Work out the finished part from the listing and answer in its coordinate system (mm). A direction names the side the tool comes from. Give positions to 0.01 mm unless a question says otherwise; leave off trailing zeros. Write each loop counter-clockwise with the first axis right and the second up, starting at its lowest first coordinate (ties: lowest second). Pieces come first, ordered by that corner, then holes. Notation, with made-up numbers: (72.25, 68.5) - (89.25, 68.5) arc R10 cw to (89.25, 74.5) - close; hole circle Ø2 at (53.25, 74.25). An arc over 180 degrees is marked (long way). Write item = value, one per line.
from build123d import *

# Parameters (mm, degrees)
F0_W     = 60
F0_H     = 30
F1_DEPTH = 30
F2_W     = 30
F2_H     = 30
F3_DEPTH = 40
F3_TAPER = 7
F4_R     = 7.1976041046
F5_DEPTH = 40


with BuildPart() as f1:
    # F0 (on Front) → F1 (new body)
    with BuildSketch(Plane.XZ):
        with Locations((-30, -15)):
            Rectangle(F0_W, F0_H)
    extrude(amount=F1_DEPTH)

    # F2 (on face) → F3 (join)
    with BuildSketch(Plane.XY):
        with Locations((-15, -15)):
            Rectangle(F2_W, F2_H)
    extrude(amount=F3_DEPTH, taper=F3_TAPER)

    # F4 (on face) → F5 (cut)
    with BuildSketch(Plane.XY.offset(40)):
        with Locations((-15, -13.6708561331)):
            Circle(F4_R)
    extrude(amount=-F5_DEPTH, mode=Mode.SUBTRACT)


solid = f1.part
1. Find section D-D, the plane x = -24. Give the vertices of the cut face in (y, z).
Solution:
outline = (-30, -30) - (0, -30) - (0, 0) - (-4.91, 40) - (-25.09, 40) - (-30, 0) - close
2. A tool of negligible diameter and unlimited length cuts with its end or side. For faces 4 (the flat face through (-45, -15, 0)), 5 (the flat face through (-15, -14, 0)), 6 (the flat face through (-2.42, -14.79, 19.72)), from which of +Z, -Z, +X, -X, +Y, -Y can it reach the whole face along a straight path? Write none if from no direction.
Solution:
face_4 = +Z, -X, +Y, -Y
face_5 = +Z
face_6 = +Z, +X, +Y, -Y
3. Given pin 1 (8 mm diameter, centred on x = -7.5, z = 31, fed in from +Y); pin 2 (2 mm diameter, centred on x = -44.5, y = -10, fed in from +Z); pin 3 (6 mm diameter, centred on y = -10, z = 30.5, fed in from +X), each flat-ended and moving along its own axis, determine where each tip first touches the part or whether it passes through.
Solution:
pin_1 = -3.32
pin_2 = 0
pin_3 = -3.38
4. Find section C-C, the plane y = -8. Give the vertices of the cut face in (x, z).
Solution:
outline = (-60, -30) - (0, -30) - (0, 0) - (-4.91, 40) - (-10.57, 40) - (-10.57, 0) - (-19.43, 0) - (-19.43, 40) - (-25.09, 40) - (-30, 0) - (-60, 0) - close
5. Find section A-A, the plane x = -15. Give the vertices of the cut face in (y, z), then the cut area to 3 significant figures.
Solution:
outline = (-30, -30) - (0, -30) - (0, 0) - (-4.91, 40) - (-6.47, 40) - (-6.47, 0) - (-20.87, 0) - (-20.87, 40) - (-25.09, 40) - (-30, 0) - close
area = 1,330 mm^2
6. For a pull along X with two mould halves and no side action, classify faces 1 (the flat face through (-30, -15, -30)), 2 (the cylindrical face through (-22.19, -13.35, 20.28)), 3 (the flat face through (-60, -15, -15)) as pulls with the +X half, pulls with the -X half, needs draft (parallel to the pull), parting line crosses it, or undercut.
Solution:
face_1 = needs draft
face_2 = undercut
face_3 = pulls with the -X half
7. Find section B-B, the plane z = 13.5. Give the vertices of the cut face in (x, y), then the cut area to 3 significant figures.
Solution:
outline = (-28.34, -28.34) - (-1.66, -28.34) - (-1.66, -1.66) - (-28.34, -1.66) - close; hole circle Ø14.4 at (-15, -13.67)
area = 549 mm^2
8. Straight lines are drawn through the part: line 1 (Z direction, x = -11.5, y = -12); line 2 (Y direction, x = -15, z = 25); line 3 (Y direction, x = -15, z = 15.5). For each, find the intervals that lie inside material, in ascending order.
Solution:
line_1 = -30 to 0
line_2 = -26.93 to -20.87, -6.47 to -3.07
line_3 = -28.1 to -20.87, -6.47 to -1.9
